Job drawing, mm, ordinate dimensions from the low corner. One solid piece. A direction names the side the tool comes from. Give positions to 0.01 mm unless a question says otherwise; leave off trailing zeros. Order: outer loops, then holes, each group sorted by start corner. A loop starts at its lowest first (then second) coordinate and runs counter-clockwise, first axis right, second up. Notation, with made-up numbers: M 87.5,-26 L 112.5,-26 A18 ccw 112.5,-17 Z; hole C 3.25,37.25 d10. An arc over 180 degrees is marked long. One line per item, written item: value. Start each with the question number.
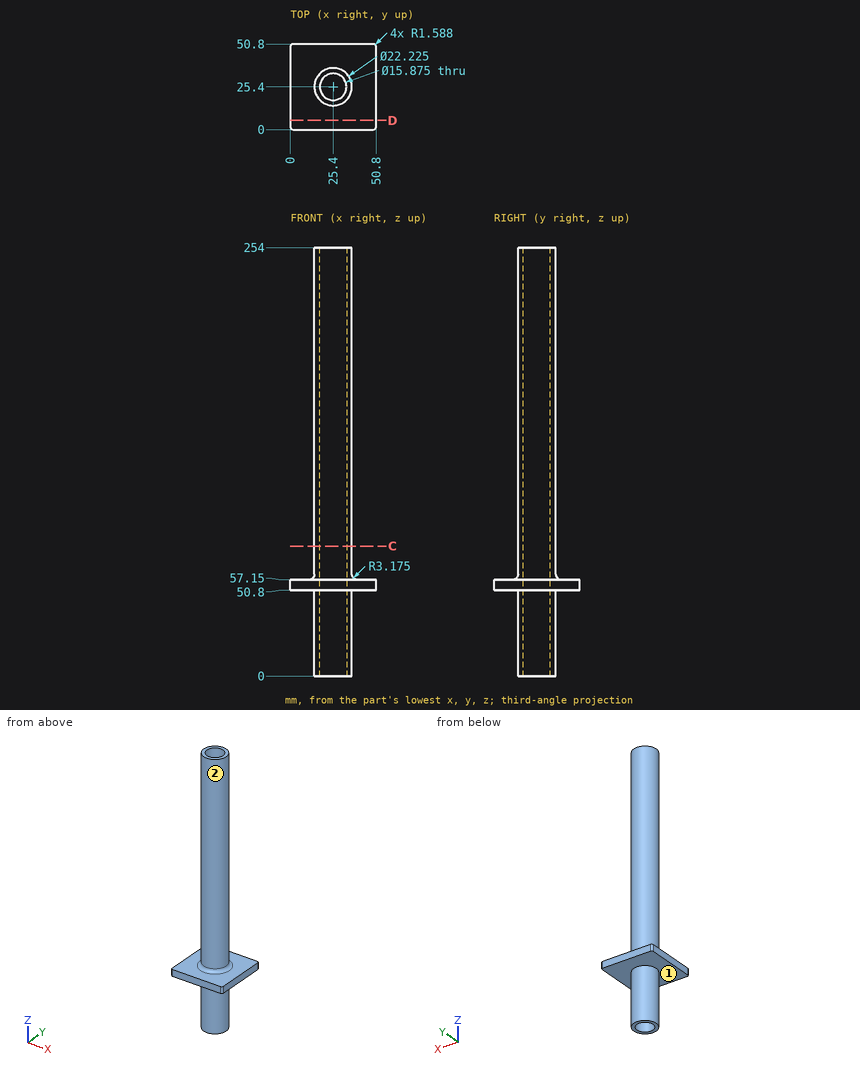
1) Slice it at C-C (z = 77). List the corners of the cut face in (x, y) (1 decimal), plus the area to 3 significant figures.
2) Tool access for the marked faces 1 and 2: list every direction of +Z, -Z, +X, -X, +Y, -Y with a clear straight run to the whole face (end or side of a thin tool).
3) Drop flat-ended pins along their axis: P1, Ø5, axis at y = 15.5, z = 80, coming from the -X side; P2, Ø5, axis at x = 20.5, z = 222.5, coming from the +Y side; P3, Ø4, axis at y = 35, z = 152, coming from the +X side; P4, Ø14.5, axis at x = 25.4, y = 25.4, coming from the +Z side. Give the stop position or say it passes through.
4) Slice it at D-D (y = 5.5). List the corners of the cut face in (x, z).
5) Drill centre lines: line 1 (X direction, y = 25, z = 97) (1 decimal); line 2 (Z direction, x = 31, y = 11). Where is each one in solid material? Low to high.
Results list:
1. outline: C 25.4,25.4 d22.2; hole C 25.4,25.4 d15.9
1. area: 190 mm²
2. face 1: -Z
2. face 2: +Z
3. P1: stops at x = 17.11
3. P2: stops at y = 36.25
3. P3: stops at x = 33.51
3. P4: passes through
4. outline: M 0,50.8 L 50.8,50.8 L 50.8,57.15 L 0,57.15 Z
5. line 1: x = 14.3 to 17.5, 33.3 to 36.5
5. line 2: z = 50.8 to 57.15
